from build123d import *

# Parameters (mm, degrees)
BOSS_EXTRUDE1_DEPTH      = 22.115
BOSS_EXTRUDE1_DEPTH_BACK = 22.115
SKETCH2_R                = 3.25
CUT_EXTRUDE1_DEPTH       = 11.115
SKETCH3_R                = 2.25
CUT_EXTRUDE2_DEPTH       = 1
SKETCH4_R                = 1.5
CUT_EXTRUDE3_DEPTH       = 6


with BuildPart() as part:
    # Sketch1 → Boss-Extrude1 (new body, two sides)
    with BuildSketch(Plane(origin=(0, 0, 0), x_dir=(0, 0, -1), z_dir=(1, 0, 0))) as boss_extrude1_sk:
        with BuildLine():
            Line((-10.25, -12.25), (23, -12.25))
            ThreePointArc((23, -12.25), (24.414213562, -12.835786438), (25, -14.25))
            Line((25, -14.25), (25, -21.25))
            ThreePointArc((25, -21.25), (25.585786438, -22.664213562), (27, -23.25))
            Line((27, -23.25), (28, -23.25))
            ThreePointArc((28, -23.25), (29.414213562, -22.664213562), (30, -21.25))
            Line((30, -21.25), (30, -14.321067812))
            ThreePointArc((30, -14.321067812), (29.886434949, -13.261467186), (29.550898606, -12.25))
            ThreePointArc((29.550898606, -12.25), (29.108985632, -11.472166783), (28.535533906, -10.785533906))
            Line((28.535533906, -10.785533906), (13.714466094, 4.035533906))
            ThreePointArc((13.714466094, 4.035533906), (12.630602337, 5.65765065), (12.25, 7.571067812))
            Line((12.25, 7.571067812), (12.25, 10.25))
            ThreePointArc((12.25, 10.25), (11.664213562, 11.664213562), (10.25, 12.25))
            Line((10.25, 12.25), (-10.25, 12.25))
            ThreePointArc((-10.25, 12.25), (-11.664213562, 11.664213562), (-12.25, 10.25))
            Line((-12.25, 10.25), (-12.25, -10.25))
            ThreePointArc((-12.25, -10.25), (-11.664213562, -11.664213562), (-10.25, -12.25))
        make_face()
        with BuildLine():
            Line((-2.375, -7.25), (-2.375, -10.5))
            Line((-2.375, -10.5), (-10.5, -10.5))
            Line((-10.5, -10.5), (-10.5, 10.5))
            Line((-10.5, 10.5), (-2.375, 10.5))
            Line((-2.375, 10.5), (-2.375, 7.25))
            ThreePointArc((-2.375, 7.25), (-1.862436867, 6.012563133), (-0.625, 5.5))
            Line((-0.625, 5.5), (0.625, 5.5))
            ThreePointArc((0.625, 5.5), (1.862436867, 6.012563133), (2.375, 7.25))
            Line((2.375, 7.25), (2.375, 10.5))
            Line((2.375, 10.5), (10.5, 10.5))
            Line((10.5, 10.5), (10.5, -10.5))
            Line((10.5, -10.5), (2.375, -10.5))
            Line((2.375, -10.5), (2.375, -7.25))
            ThreePointArc((2.375, -7.25), (1.862436867, -6.012563133), (0.625, -5.5))
            Line((0.625, -5.5), (-0.625, -5.5))
            ThreePointArc((-0.625, -5.5), (-1.862436867, -6.012563133), (-2.375, -7.25))
        make_face(mode=Mode.SUBTRACT)
    extrude(amount=BOSS_EXTRUDE1_DEPTH)
    extrude(boss_extrude1_sk.sketch, amount=-BOSS_EXTRUDE1_DEPTH_BACK)

    # Sketch2 → Cut-Extrude1 (cut)
    with BuildSketch(Plane.XY.offset(12.25)):
        Circle(SKETCH2_R)
    extrude(amount=-CUT_EXTRUDE1_DEPTH, mode=Mode.SUBTRACT)

    # Sketch3 → Cut-Extrude2 (cut)
    with BuildSketch(Plane.XY.offset(-25)):
        with Locations((14.615, -17.75)):
            Circle(SKETCH3_R)
        with Locations((-5.385, -17.75)):
            Circle(SKETCH3_R)
    extrude(amount=-CUT_EXTRUDE2_DEPTH, mode=Mode.SUBTRACT)

    # Sketch4 → Cut-Extrude3 (cut)
    with BuildSketch(Plane.XY.offset(-26)):
        with Locations((-5.385, -17.75)):
            Circle(SKETCH4_R)
        with Locations((14.615, -17.75)):
            Circle(SKETCH4_R)
    extrude(amount=-CUT_EXTRUDE3_DEPTH, mode=Mode.SUBTRACT)


solid = part.part
Could you check a few things on this model? Use its own coordinates, in mm. A direction names the side the tool comes from. Give positions to 0.01 mm unless a question says otherwise; leave off trailing zeros. Write each loop counter-clockwise with the first axis right and the second up, starting at its lowest first coordinate (ties: lowest second). Pieces come first, ordered by that corner, then holes. Notation, with made-up numbers: (-21.5, -37) -> (0.5, -37) arc R8 ccw to (0.5, -33) -> close; hole circle Ø9 at (-20.75, 80). An arc over 180 degrees is marked (long way). Answer as a JSON object with one key per item and string values.
Q1. Which directions (+Z, -Z, +X, -X, +Y, -Y) give clear straight access to the entire face, cutting with the end or side of a thin tool? Please do faces 4 (the cylindrical face through (0.31, 6, -1.85)), 5 (the flat face through (0, -18, -25)), 6 (the flat face through (15, -16, -26)).
Taken from the geometry:
{"face 4": "+X, -X", "face 5": "+Z, +X, -X, -Y", "face 6": "+Z"}
Q2. Please list where these lines run through material, in increasing order: L1, parallel to Z at x = -3, y = 8.5 (3 decimals); L2, parallel to Z at x = 12.5, y = -10 (3 decimals); L3, parallel to Z at x = 10, y = -18.
Taken from the geometry:
{"L1": "z = -12.25 to -10.5, -2.375 to 2.375, 10.5 to 12.25", "L2": "z = -27.75 to -10.5, -2.375 to 2.375, 10.5 to 12.25", "L3": "z = -30 to -25"}
Q3. Suppose I cut it at D-D on y = -17.75. Write out the boundary of the cut face in (x, z) (3 decimals).
Taken from the geometry:
{"outline": "(-22.115, -30) -> (-6.885, -30) -> (-6.885, -26) -> (-7.635, -26) -> (-7.635, -25) -> (-22.115, -25) -> close; (-3.885, -30) -> (13.115, -30) -> (13.115, -26) -> (12.365, -26) -> (12.365, -25) -> (-3.135, -25) -> (-3.135, -26) -> (-3.885, -26) -> close; (16.115, -30) -> (22.115, -30) -> (22.115, -25) -> (16.865, -25) -> (16.865, -26) -> (16.115, -26) -> close"}
Q4. We'd pull the mould along Z, two halves only. Please class faces 1 (the cylindrical face through (-2.579, -1.978, 11.387)), 2 (the flat face through (-5, -16, -26)), 3 (the flat face through (0, -5, 10.5)): released by +Z, released by -Z, zero draft, split by the parting line, or undercut.
Taken from the geometry:
{"face 1": "zero draft", "face 2": "released by +Z", "face 3": "undercut"}
Q5. Will these pins go through, and if not, where does the flat tip stop? pin 1 Ø10 at (x, z) = (17, -20.5) entering from -Y; pin 2 Ø5 at (x, y) = (-6, -17.5) entering from +Z; pin 3 Ø2.5 at (x, y) = (-5.385, -17.75) entering from -Z (3 decimals); pin 4 Ø10 at (y, z) = (-14, -19) entering from +X (3 decimals).
Taken from the geometry:
{"pin 1": "stops at y = -22.57", "pin 2": "stops at z = -25", "pin 3": "passes through", "pin 4": "stops at x = 22.115"}
Q6. Suppose I cut it at A-A on y = 0. Write out the boundary of the cut face in (x, z) (3 decimals), then the cut area to 3 significant figures.
Taken from the geometry:
{"outline": "(-22.115, -17.75) -> (22.115, -17.75) -> (22.115, -10.5) -> (-22.115, -10.5) -> close; (-22.115, 10.5) -> (-3.25, 10.5) -> (-3.25, 12.25) -> (-22.115, 12.25) -> close; (3.25, 10.5) -> (22.115, 10.5) -> (22.115, 12.25) -> (3.25, 12.25) -> close", "area": "387 mm²"}
Q7. Suppose I cut it at C-C on z = -6. Write out the boundary of the cut face in (x, y) (3 decimals), then the cut area to 3 significant figures.
Taken from the geometry:
{"outline": "(-22.115, -12.25) -> (22.115, -12.25) -> (22.115, -10.5) -> (-22.115, -10.5) -> close; (-22.115, 10.5) -> (22.115, 10.5) -> (22.115, 12.25) -> (-22.115, 12.25) -> close", "area": "155 mm²"}
